Could you check a few things on this drawing? It's one solid part, dimensions in mm from its lowest x, y, z. Round coordinates to 2 decimals unless told otherwise and drop trailing zeros. Loops run counter-clockwise (first coordinate to the right, second up) from the corner with the lowest first, then second, coordinate; pieces in that order, holes last. Notation, with made-up numbers: (-6, 19.5) -> (12, 19.5) arc R12 cw to (12, 26.5) -> close; hole circle Ø3 at (80, -18). An arc over 180 degrees is marked (long way). Write each question's results on one line, items separated by ' | '.
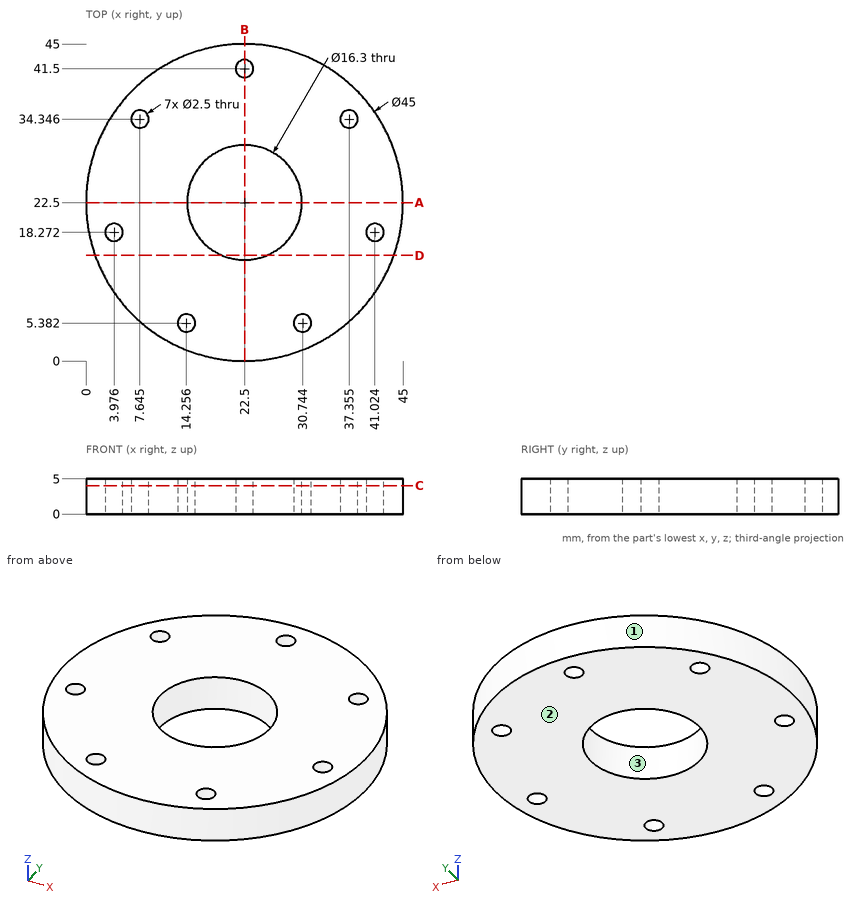
1) I want a section at C-C, the plane z = 4.05. Give the number of separate pieces and of enclosed holes in the cut face, plus the area to 3 significant figures.
Model answer:
separate pieces: 1 | enclosed holes: 8 | area: 1,350 mm2
2) I want a section at A-A, the plane y = 22.5. Write out the boundary of the cut face in (x, z).
Model answer:
outline: (0, 0) -> (14.35, 0) -> (14.35, 5) -> (0, 5) -> close; (30.65, 0) -> (45, 0) -> (45, 5) -> (30.65, 5) -> close
3) I want a section at B-B, the plane x = 22.5. Write out the boundary of the cut face in (y, z), plus the area to 3 significant figures.
Model answer:
outline: (0, 0) -> (14.35, 0) -> (14.35, 5) -> (0, 5) -> close; (30.65, 0) -> (40.25, 0) -> (40.25, 5) -> (30.65, 5) -> close; (42.75, 0) -> (45, 0) -> (45, 5) -> (42.75, 5) -> close | area: 131 mm2
4) I want a section at D-D, the plane y = 15. Write out the boundary of the cut face in (x, z), plus the area to 3 significant figures.
Model answer:
outline: (1.29, 0) -> (19.31, 0) -> (19.31, 5) -> (1.29, 5) -> close; (25.69, 0) -> (43.71, 0) -> (43.71, 5) -> (25.69, 5) -> close | area: 180 mm2
5) I'm going to push flat-ended pins straight in: pin 1 (2 mm diameter, centred on x = 13, z = 2, fed in from -Y); pin 2 (2 mm diameter, centred on x = 14.26, y = 5.38, fed in from -Z); pin 3 (3 mm diameter, centred on x = 37, z = 3.5, fed in from -Y) (1 decimal). Where does each tip first touch, or does it pass through?
Model answer:
pin 1: stops at y = 1.67 | pin 2: passes through | pin 3: stops at y = 4.1
6) I need wall thicknesses on line 1 (X direction, y = 18, z = 4.55) (1 decimal); line 2 (Y direction, x = 7, z = 1.5) (1 decimal); line 3 (Y direction, x = 24, z = 0.7). Which ranges of each line are inside material? Lowest first, please.
Model answer:
line 1: x = 0.5 to 2.8, 5.2 to 15.7, 29.3 to 39.8, 42.2 to 44.5 | line 2: y = 6.2 to 33.3, 35.4 to 38.8 | line 3: y = 0.05 to 14.49, 30.51 to 44.95
7) If we mould it in two halves opening along X, with no side actions, what happens to the marked faces 1, 2 and 3? For each: released by +X, released by -X, zero draft, split by the parting line, or undercut.
Model answer:
face 1: split by the parting line | face 2: zero draft | face 3: undercut
